Verification items for the finished model (mm, model axes). Face numbers are marked on the shaded views. A direction names the side the tool comes from. Give positions to 0.01 mm unless a question says otherwise; leave off trailing zeros. Order: outer loops, then holes, each group sorted by start corner. A loop starts at its lowest first (then second) coordinate and runs counter-clockwise, first axis right, second up. Notation, with made-up numbers: (3, 30) -> (48, 30) arc R20 ccw to (48, 52) -> close; hole circle Ø7 at (-32, 60). An arc over 180 degrees is marked (long way). Write each question's results on one line, items separated by ' | '. Start each with the question number.
1. Cross-section at C-C, the plane z = 2. State how many separate pieces and enclosed holes the cut face has, then the cut area to 3 significant figures.
2. Cross-section at D-D, the plane x = -6.75. Enter the section's corners in (y, z), then the cut area to 3 significant figures.
3. Material ranges on L1, parallel to Y at x = 0, z = 1.75; L2, parallel to Y at x = -7, z = 2; L3, parallel to X at y = 10.75, z = 3.5 (3 decimals), recorded low to high. Write a range as from..to.
4. Depth check by flat-ended pin: pin 1 Ø1 at (y, z) = (-11, 4) entering from -X; pin 2 Ø1.5 at (x, z) = (-2.5, 3) entering from +Y; pin 3 Ø2 at (x, y) = (-9.9, 3.22) entering from -Z (3 decimals); pin 4 Ø3 at (x, z) = (-3, 2) entering from -Y. Enter the tip coordinate at first touch or a pass-through.
5. Cross-section at A-A, the plane x = 0. Enter the section's corners in (y, z), then the cut area to 3 significant figures.
6. Set-up check for the marked faces 4, 5 and 6: record each of +Z, -Z, +X, -X, +Y, -Y from which the full face is reachable in a straight line by a thin tool's end or side.
7. Cross-section at B-B, the plane x = 6. Enter the section's corners in (y, z), then the cut area to 3 significant figures.
8. Mould release check, pull along Y, two halves, no side actions. Record for the marked faces 1, 2 and 3: +Y half, -Y half, draft (parallel to the pull), parting line (faces both ways), or undercut.
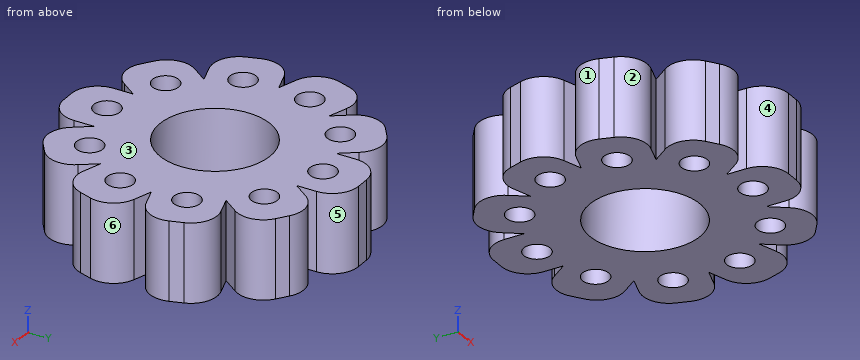
from build123d import *

# Parameters (mm, degrees)
F0_R     = 7.62
F0_R_2   = 5.334
F1_DEPTH = 7.62
F2_R     = 1.27
F3_DEPTH = 7.62
F4_R     = 2.54
F5_COUNT = 10


with BuildPart() as f1:
    # F0 (on Top) → F1 (new body)
    with BuildSketch(Plane.XY):
        Circle(F0_R)
        Circle(F0_R_2, mode=Mode.SUBTRACT)
    extrude(amount=F1_DEPTH)

    # F2 (on face) → F3 (join)
    with BuildSketch(Plane.XY.offset(7.62)):
        with BuildLine():
            ThreePointArc((-3.175, 6.927032), (0, 7.62), (3.175, 6.927032))
            Line((3.175, 6.927032), (3.175, 14.224))
            Line((3.175, 14.224), (-3.175, 14.224))
            Line((-3.175, 14.224), (-3.175, 6.927032))
        make_face()
        with Locations((0, 10.414)):
            Circle(F2_R, mode=Mode.SUBTRACT)
    extrude(amount=-F3_DEPTH)

    # F4
    f4_edges = [f1.edges().sort_by_distance(p)[0] for p in [
        (3.175, 14.224, 3.81),
        (-3.175, 14.224, 3.81),
    ]]
    fillet(f4_edges, radius=F4_R)

    # F5: F1 ×10 about axis
    f5_axis = Axis((0, 0, 0), (0, 0, 1))


with BuildPart() as f1_1:
    add(f1.part)
    for i in range(1, F5_COUNT):
        add(f1.part.rotate(f5_axis, i * 360 / F5_COUNT))


solid = f1_1.part
Results below:
1) separate pieces: 1 | enclosed holes: 11 | area: 425 mm²
2) outline: (-12.33, 0) -> (-9.53, 0) -> (-9.53, 7.62) -> (-12.33, 7.62) -> close; (-7.32, 0) -> (7.32, 0) -> (7.32, 7.62) -> (-7.32, 7.62) -> close; (9.53, 0) -> (12.33, 0) -> (12.33, 7.62) -> (9.53, 7.62) -> close | area: 154 mm²
3) L1: y = -14.22..-11.68, -9.14..-5.33, 5.33..9.14, 11.68..14.22 | L2: y = -12.28..-9.34, -7.51..7.51, 9.34..12.28 | L3: x = -9.295..-3.886, -3.175..-1.225, 1.225..3.175, 3.886..9.295
4) pin 1: stops at x = -9.49 | pin 2: stops at y = 13.97 | pin 3: passes through | pin 4: stops at y = -14.07
5) outline: (-14.22, 0) -> (-11.68, 0) -> (-11.68, 7.62) -> (-14.22, 7.62) -> close; (-9.14, 0) -> (-5.33, 0) -> (-5.33, 7.62) -> (-9.14, 7.62) -> close; (5.33, 0) -> (9.14, 0) -> (9.14, 7.62) -> (5.33, 7.62) -> close; (11.68, 0) -> (14.22, 0) -> (14.22, 7.62) -> (11.68, 7.62) -> close | area: 96.8 mm²
6) face 4: +Z, -Z, -Y | face 5: +Z, -Z, +Y | face 6: +Z, -Z, +X
7) outline: (-12.34, 0) -> (-9.69, 0) -> (-9.69, 7.62) -> (-12.34, 7.62) -> close; (-7.16, 0) -> (7.16, 0) -> (7.16, 7.62) -> (-7.16, 7.62) -> close; (9.69, 0) -> (12.34, 0) -> (12.34, 7.62) -> (9.69, 7.62) -> close | area: 150 mm²
8) face 1: undercut | face 2: -Y half | face 3: draft
